Geometry: see drawing. Coordinates: mm, zero at the bounding-box minimum. A direction names the side the tool comes from. Round coordinates to 2 decimals unless told otherwise and drop trailing zeros. Order: outer loops, then holes, each group sorted by start corner. A loop starts at its lowest first (then second) coordinate and runs counter-clockwise, first axis right, second up. Notation, with made-up numbers: (49.25, 53) -> (97.25, 53) arc R29 ccw to (97.25, 83) -> close; hole circle Ø7 at (42, 51.5). An arc over 180 degrees is marked (long way). Put each result on its own line as item: value.
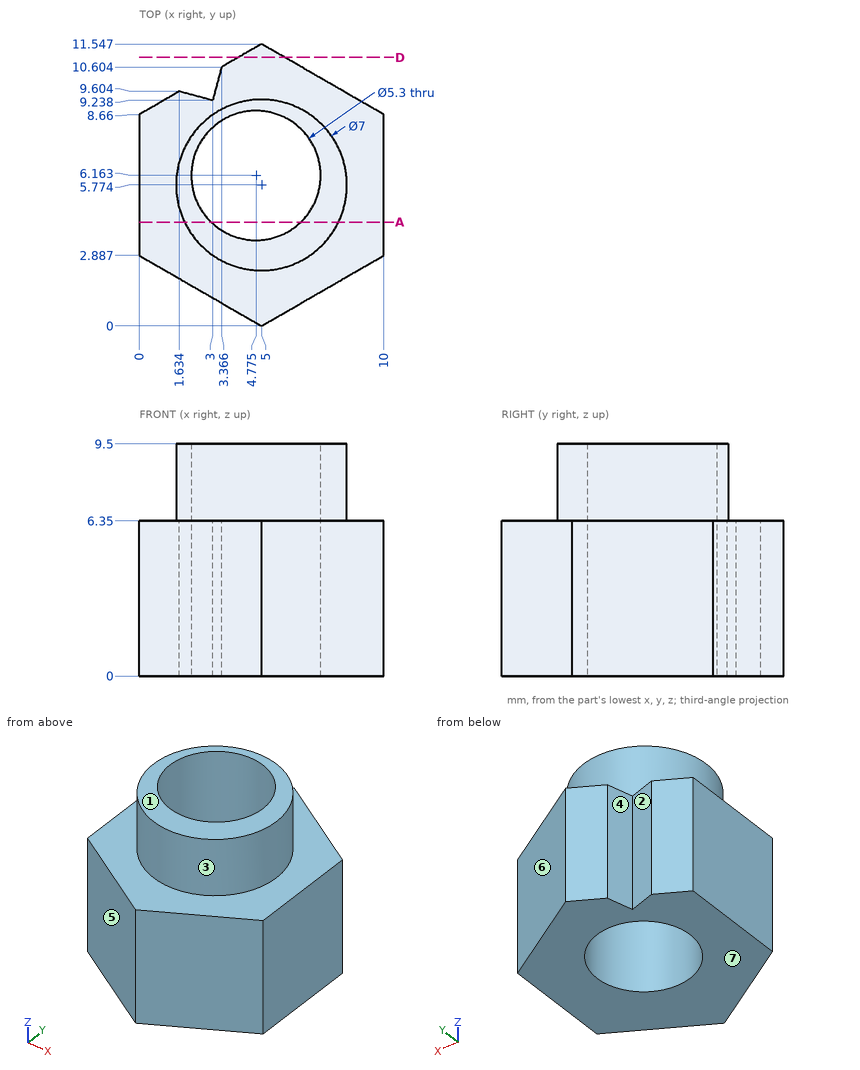
1. Set-up query: the marked faces 1, 2 and 3. Return all of +Z, -Z, +X, -X, +Y, -Y with unobstructed straight access to the full face (end or side cutting, diameter ignored); none if empty.
Ans:
face 1: +Z, +X, -X, +Y, -Y
face 2: +Z, -Z, +Y
face 3: +Z
2. Cut plane D-D on y = 11. Return loops of the section in (x, z).
Ans:
outline: (4.05, 0) -> (5.95, 0) -> (5.95, 6.35) -> (4.05, 6.35) -> close
3. Cut plane A-A on y = 4.25. Return loops of the section in (x, z).
Ans:
outline: (0, 0) -> (2.94, 0) -> (2.94, 9.5) -> (1.85, 9.5) -> (1.85, 6.35) -> (0, 6.35) -> close; (6.61, 0) -> (10, 0) -> (10, 6.35) -> (8.15, 6.35) -> (8.15, 9.5) -> (6.61, 9.5) -> close
4. Material intervals for probe 1 along Z at (x, y) = (1, 6.5); probe 2 along Y at (x, z) = (6, 6.5) (1 decimal); probe 3 along Y at (x, z) = (4.75, 9) (1 decimal), sorted ascending.
Ans:
probe 1: 0 to 6.35
probe 2: 2.4 to 3.8, 8.5 to 9.1
probe 3: 2.3 to 3.5, 8.8 to 9.3
5. Contact query for flat-ended pins moving along their axis: P1, Ø1.5, axis at x = 7.5, y = 3.5, coming from the -Z side; P2, Ø3, axis at x = 2, z = 2, coming from the -Y side (1 decimal); P3, Ø4, axis at x = 2, z = 3, coming from the +Y side. Output: stop coordinate, or through.
Ans:
P1: z = 0
P2: y = 0.9
P3: y = 10.97
6. Draft query along X for the marked faces 4, 5, 6 and 7. Return one class per face: +X half, -X half, draft (parallel to the pull), parting line (faces both ways), or undercut.
Ans:
face 4: undercut
face 5: -X half
face 6: +X half
face 7: draft
